Geometry: final body of the model. Coordinates: model frame, mm. Give positions to 0.01 mm unless a question says otherwise; leave off trailing zeros. Order: outer loops, then holes, each group sorted by start corner. A loop starts at its lowest first (then second) coordinate and runs counter-clockwise, first axis right, second up. Notation, with made-up numbers: (-8.5, 0) -> (24.5, 0) arc R7 ccw to (24.5, 5) -> close; hole circle Ø8 at (-16, 78). An arc over 180 degrees is marked (long way). One line per question, with ' | ' between items. Start each with the question number.
(1) First-contact query: pin 1 Ø1.5 at (y, z) = (-8, 3.5) entering from +X; pin 2 Ø1.4 at (x, y) = (45, 12) entering from -Z; pin 3 Ø2.5 at (x, z) = (-29.5, 2) entering from -Y. Flat tips, straight axial feed; report the tip coordinate or a pass-through.
(2) Section D-D (y = 13.5). Return loops of the section in (x, z).
(3) Section C-C (x = 18). Return loops of the section in (y, z), then the cut area to 3 significant figures.
(4) Ray query, L1, parallel to Y at x = 30.5, z = 1.5; L2, parallel to X at y = -12, z = 1; L3, parallel to Z at x = -12.5, y = 4. Return the intervals inside material, ascending.
(5) Section B-B (z = 1.5). Return loops of the section in (x, y) (3 decimals), then the cut area to 3 significant figures.
(6) Section A-A (y = -7.5). Return loops of the section in (x, z).
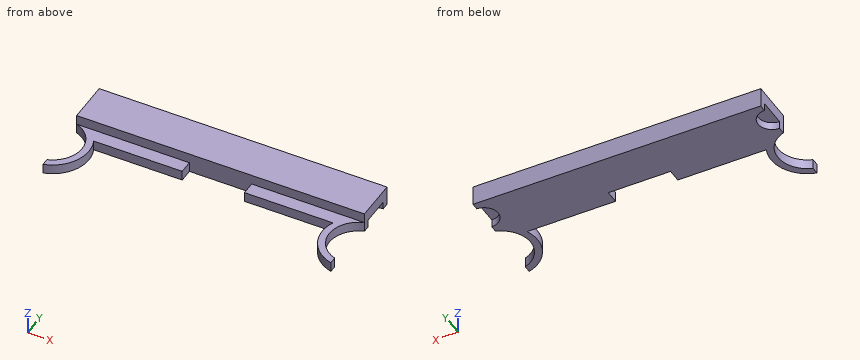
```python
from build123d import *

# Parameters (mm, degrees)
F1_DEPTH = 6.477
F2_DEPTH = 3.2512
F4_DEPTH = 2.54


with BuildPart() as f1:
    # F0 (on Top) → F1 (new body)
    with BuildSketch(Plane.XY):
        Polygon((46.99, 18.161), (-46.99, 18.161), (-46.99, 4.401166), (-10.16, 4.401166), (10.16, 4.401166), (46.99, 4.401166), align=None)
    extrude(amount=F1_DEPTH)

    # F0 (on Top) → F2 (join)
    with BuildSketch(Plane.XY):
        with BuildLine():
            Line((-10.16, 4.401166), (-46.99, 4.401166))
            ThreePointArc((-46.99, 4.401166), (-40.386, -4.664891), (-46.99, -13.730948))
            Line((-46.99, -13.730948), (-46.99, -16.108993))
            ThreePointArc((-46.99, -16.108993), (-39.314297, -9.881174), (-39.060262, 0))
            Line((-39.060262, 0), (-10.16, 0))
            Line((-10.16, 0), (-10.16, 4.401166))
        make_face()
        with BuildLine():
            ThreePointArc((46.99, -13.730948), (40.386, -4.664891), (46.99, 4.401166))
            Line((46.99, 4.401166), (10.16, 4.401166))
            Line((10.16, 4.401166), (10.16, 0))
            Line((10.16, 0), (39.060262, 0))
            ThreePointArc((39.060262, 0), (39.314297, -9.881174), (46.99, -16.108993))
            Line((46.99, -16.108993), (46.99, -13.730948))
        make_face()
    extrude(amount=F2_DEPTH)

    # F3 (on face) → F4 (cut)
    with BuildSketch(Plane.XY):
        with BuildLine():
            Line((-46.99, 15.853083), (-46.99, 6.709083))
            ThreePointArc((-46.99, 6.709083), (-42.418, 11.281083), (-46.99, 15.853083))
        make_face()
        with BuildLine():
            ThreePointArc((46.99, 15.853083), (42.418, 11.281083), (46.99, 6.709083))
            Line((46.99, 6.709083), (46.99, 15.853083))
        make_face()
    extrude(amount=F4_DEPTH, mode=Mode.SUBTRACT)


solid = f1.part
```
Response:
1) pin 1: stops at x = 41.29 | pin 2: stops at z = 2.54 | pin 3: stops at y = 0
2) outline: (-46.99, 2.54) -> (-42.99, 2.54) -> (-42.99, 0) -> (42.99, 0) -> (42.99, 2.54) -> (46.99, 2.54) -> (46.99, 6.48) -> (-46.99, 6.48) -> close
3) outline: (0, 0) -> (18.16, 0) -> (18.16, 6.48) -> (4.4, 6.48) -> (4.4, 3.25) -> (0, 3.25) -> close | area: 103 mm^2
4) L1: y = 0 to 18.16 | L2: x = -43.83 to -40.65, 40.65 to 43.83 | L3: z = 0 to 3.25
5) outline: (-46.99, -16.109) arc R11.811 ccw to (-39.06, 0) -> (-10.16, 0) -> (-10.16, 4.401) -> (10.16, 4.401) -> (10.16, 0) -> (39.06, 0) arc R11.811 ccw to (46.99, -16.109) -> (46.99, -13.731) arc R9.525 cw to (46.99, 4.401) -> (46.99, 6.709) arc R4.572 cw to (46.99, 15.853) -> (46.99, 18.161) -> (-46.99, 18.161) -> (-46.99, 15.853) arc R4.572 cw to (-46.99, 6.709) -> (-46.99, 4.401) arc R9.525 cw to (-46.99, -13.731) -> close | area: 1,610 mm^2
6) outline: (-40.82, 0) -> (-38.45, 0) -> (-38.45, 3.25) -> (-40.82, 3.25) -> close; (38.45, 0) -> (40.82, 0) -> (40.82, 3.25) -> (38.45, 3.25) -> close
